Read the model definition and answer for the solid it produces. Units are mm, in the model's axes. A direction names the side the tool comes from. Coordinates: 2 decimals unless noted, no trailing zeros. Order: outer loops, then holes, each group sorted by start corner. A loop starts at its lowest first (then second) coordinate and runs counter-clockwise, first axis right, second up. Notation, with made-up numbers: (9, 38) -> (46, 38) arc R28 ccw to (46, 77) -> close; hole circle Ø2 at (49.5, 55.25). An arc over 180 degrees is marked (long way). Answer in a Markdown table with one row per item.
from build123d import *

# Parameters (mm, degrees)
SKETCH1_R           = 25.4
SKETCH1_R_2         = 2.54
SKETCH1_R_3         = 3.2639
BOSS_EXTRUDE1_DEPTH = 6.35
SKETCH2_R           = 25.4
CUT_EXTRUDE1_DEPTH  = 10


with BuildPart() as part:
    # Sketch1 → Boss-Extrude1 (new body)
    with BuildSketch(Plane(origin=(0, 0, 0), x_dir=(1, 0, 0), z_dir=(0, 1, 0))):
        with Locations(Location((0, 0, 0), (0, 0, 270))):
            Circle(SKETCH1_R)
        with Locations(Location((0, 0, 0), (0, 0, 270))):
            Circle(SKETCH1_R_2, mode=Mode.SUBTRACT)
        with Locations(Location((0, 12.7, 0), (0, 0, 270))):
            Circle(SKETCH1_R_3, mode=Mode.SUBTRACT)
        with Locations(Location((12.7, 0, 0), (0, 0, 270))):
            Circle(SKETCH1_R_3, mode=Mode.SUBTRACT)
        with Locations(Location((0, -12.7, 0), (0, 0, 270))):
            Circle(SKETCH1_R_3, mode=Mode.SUBTRACT)
        with Locations(Location((-12.7, 0, 0), (0, 0, 270))):
            Circle(SKETCH1_R_3, mode=Mode.SUBTRACT)
    extrude(amount=BOSS_EXTRUDE1_DEPTH)

    # Sketch2 → Cut-Extrude1 (cut)
    with BuildSketch(Plane(origin=(0, 0, 0), x_dir=(1, 0, 0), z_dir=(0, 1, 0))):
        Circle(SKETCH2_R)
        with BuildLine():
            ThreePointArc((-4.7625, 12.7), (0, 17.4625), (4.7625, 12.7))
            Line((4.7625, 12.7), (4.7625, 6.7625))
            ThreePointArc((4.7625, 6.7625), (5.348286438, 5.348286438), (6.7625, 4.7625))
            Line((6.7625, 4.7625), (12.7, 4.7625))
            ThreePointArc((12.7, 4.7625), (16.067596045, 3.367596045), (17.4625, 0))
            ThreePointArc((17.4625, 0), (16.067596045, -3.367596045), (12.7, -4.7625))
            Line((12.7, -4.7625), (6.7625, -4.7625))
            ThreePointArc((6.7625, -4.7625), (5.348286438, -5.348286438), (4.7625, -6.7625))
            Line((4.7625, -6.7625), (4.7625, -12.7))
            ThreePointArc((4.7625, -12.7), (0, -17.4625), (-4.7625, -12.7))
            Line((-4.7625, -12.7), (-4.7625, -6.7625))
            ThreePointArc((-4.7625, -6.7625), (-5.348286438, -5.348286438), (-6.7625, -4.7625))
            Line((-6.7625, -4.7625), (-12.7, -4.7625))
            ThreePointArc((-12.7, -4.7625), (-17.4625, 0), (-12.7, 4.7625))
            Line((-12.7, 4.7625), (-6.7625, 4.7625))
            ThreePointArc((-6.7625, 4.7625), (-5.348286438, 5.348286438), (-4.7625, 6.7625))
            Line((-4.7625, 6.7625), (-4.7625, 12.7))
        make_face(mode=Mode.SUBTRACT)
    extrude(amount=CUT_EXTRUDE1_DEPTH, mode=Mode.SUBTRACT)


solid = part.part
Q1. For faces 5 (the face through (10, 3, 4.762)), 6 (the face through (-17.46, 3.13, 0.1)), 7 (the face through (10, 3, -4.762)), determine the directions among +Z, -Z, +X, -X, +Y, -Y from which every point of the face is accessible in a straight line to the end or side of a thin tool.
Outcome:
| item | result |
|---|---|
| face 5 | +Z, +X, +Y, -Y |
| face 6 | -X, +Y, -Y |
| face 7 | -Z, +X, +Y, -Y |
Q2. The part is cut by section C-C (z = 11). Write down the section's boundary in (x, y), then the cut area to 3 significant figures.
Outcome:
| item | result |
|---|---|
| outline | (-4.76, 0) -> (-2.79, 0) -> (-2.79, 6.35) -> (-4.76, 6.35) -> close; (2.79, 0) -> (4.76, 0) -> (4.76, 6.35) -> (2.79, 6.35) -> close |
| area | 25.1 mm² |
Q3. The part is cut by section A-A (x = 0). Write down the section's boundary in (y, z).
Outcome:
| item | result |
|---|---|
| outline | (0, -17.46) -> (6.35, -17.46) -> (6.35, -15.96) -> (0, -15.96) -> close; (0, -9.44) -> (6.35, -9.44) -> (6.35, -2.54) -> (0, -2.54) -> close; (0, 2.54) -> (6.35, 2.54) -> (6.35, 9.44) -> (0, 9.44) -> close; (0, 15.96) -> (6.35, 15.96) -> (6.35, 17.46) -> (0, 17.46) -> close |
Q4. The part is cut by section D-D (x = 15). Write down the section's boundary in (y, z), then the cut area to 3 significant figures.
Outcome:
| item | result |
|---|---|
| outline | (0, -4.17) -> (6.35, -4.17) -> (6.35, -2.32) -> (0, -2.32) -> close; (0, 2.32) -> (6.35, 2.32) -> (6.35, 4.17) -> (0, 4.17) -> close |
| area | 23.6 mm² |
Q5. Consider line 1 (Z direction, x = 2, y = 0.75); line 2 (Z direction, x = 1.5, y = 1.5); line 3 (X direction, y = 3.25, z = 12.7). Determine where each line is inside the solid, lowest interval first.
Outcome:
| item | result |
|---|---|
| line 1 | -17.02 to -15.28, -10.12 to -1.57, 1.57 to 10.12, 15.28 to 17.02 |
| line 2 | -17.22 to -15.6, -9.8 to -2.05, 2.05 to 9.8, 15.6 to 17.22 |
| line 3 | -4.76 to -3.26, 3.26 to 4.76 |
Q6. For a pull along Z with two mould halves and no side action, classify faces 1 (the face through (-4.762, 3, -10)), 2 (the face through (9.514, 3.131, -0.708)), 3 (the face through (0.14, 3.13, 9.44)), 4 (the face through (-10, 3, -4.762)) as pulls with the +Z half, pulls with the -Z half, needs draft (parallel to the pull), parting line crosses it, or undercut.
Outcome:
| item | result |
|---|---|
| face 1 | needs draft |
| face 2 | undercut |
| face 3 | undercut |
| face 4 | pulls with the -Z half |
Q7. The part is cut by section B-B (y = 1.75). Write down the section's boundary in (x, z) (1 decimal), then the cut area to 3 significant figures.
Outcome:
| item | result |
|---|---|
| outline | (-12.7, -4.8) -> (-6.8, -4.8) arc R2 cw to (-4.8, -6.8) -> (-4.8, -12.7) arc R4.8 ccw to (4.8, -12.7) -> (4.8, -6.8) arc R2 cw to (6.8, -4.8) -> (12.7, -4.8) arc R4.8 ccw to (12.7, 4.8) -> (6.8, 4.8) arc R2 cw to (4.8, 6.8) -> (4.8, 12.7) arc R4.8 ccw to (-4.8, 12.7) -> (-4.8, 6.8) arc R2 cw to (-6.8, 4.8) -> (-12.7, 4.8) arc R4.8 ccw to start; hole circle Ø6.5 at (-12.7, 0); hole circle Ø6.5 at (0, -12.7); hole circle Ø6.5 at (0, 12.7); hole circle Ø5.1 at (0, 0); hole circle Ø6.5 at (12.7, 0) |
| area | 385 mm² |
Q8. Given pin 1 (1.8 mm diameter, centred on y = 3, z = -11, fed in from -X); pin 2 (3 mm diameter, centred on y = 4, z = -8.5, fed in from +X); pin 3 (1.8 mm diameter, centred on x = 8.5, y = 4, fed in from -Z), each flat-ended and moving along its own axis, determine where each tip first touches the part or whether it passes through.
Outcome:
| item | result |
|---|---|
| pin 1 | x = -4.76 |
| pin 2 | x = 4.76 |
| pin 3 | z = -4.76 |
